```python
from build123d import *

# Parameters (mm, degrees)
F0_W     = 78.25
F0_H     = 40
F1_DEPTH = 2
F3_DEPTH = 77.25


with BuildPart() as f1:
    # F0 (on Top) → F1 (new body)
    with BuildSketch(Plane.XY):
        Rectangle(F0_W, F0_H)
    extrude(amount=F1_DEPTH)

    # F2 (on face) → F3 (cut)
    with BuildSketch(Plane(origin=(-39.125, 0, 0), x_dir=(0, -1, 0), z_dir=(-1, 0, 0))):
        Polygon((18, 2), (-18, 2), (-19, 0), (19, 0), align=None)
    extrude(amount=-F3_DEPTH, mode=Mode.SUBTRACT)


solid = f1.part
```
The listing builds one solid part. Answer for the finished solid, in the listing's coordinates (mm). A direction names the side the tool comes from. Give positions to 0.01 mm unless a question says otherwise; leave off trailing zeros. Order: outer loops, then holes, each group sorted by start corner. A loop starts at its lowest first (then second) coordinate and runs counter-clockwise, first axis right, second up. Notation, with made-up numbers: (20.5, 48.25) - (40.5, 48.25) arc R21 ccw to (40.5, 53.25) - close; hole circle Ø9 at (83, -28.5). An arc over 180 degrees is marked (long way). Answer in a Markdown table with one row per item. Add a question column.
Q1. For a pull along Y with two mould halves and no side action, classify faces 1 (the flat face through (38.125, 0, 1)), 2 (the flat face through (-1, -20, 1)), 3 (the flat face through (-0.2, 19.4, 0)), 4 (the flat face through (-1, -18.5, 1)) as released by +Y, released by -Y, zero draft, split by the parting line, or undercut.
Q2. The part is cut by section A-A (x = 6.5). Determine the outline of the cut face in (y, z).
Q3. Which of the six approach directions +Z, -Z, +X, -X, +Y, -Y give full straight-line access (tool end or side, diameter ignored) to faces 5 (the flat face through (-1, 18.5, 1)), 6 (the flat face through (-1, 20, 1))?
Q4. Find the intervals of material crossed by line 1 along X through (y, z) = (15.5, 1.7) (3 decimals); line 2 along Y through (x, z) = (-14, 1); line 3 along Y through (x, z) = (9, 0.6), in increasing order. Write a range as [from, to].
Q5. The part is cut by section B-B (z = 0.6). Determine the outline of the cut face in (x, y) (3 decimals), then the cut area to 3 significant figures.
Q6. The part is cut by section C-C (y = -4). Determine the outline of the cut face in (x, z) (3 decimals).
Determined:
| question | item | result |
|---|---|---|
| 1 | face 1 | undercut |
| 1 | face 2 | released by -Y |
| 1 | face 3 | zero draft |
| 1 | face 4 | undercut |
| 2 | outline | (-20, 0) - (-19, 0) - (-18, 2) - (-20, 2) - close; (18, 2) - (19, 0) - (20, 0) - (20, 2) - close |
| 3 | face 5 | -Z, -X |
| 3 | face 6 | +Z, -Z, +X, -X, +Y |
| 4 | line 1 | x = [38.125, 39.125] |
| 4 | line 2 | y = [-20, -18.5], [18.5, 20] |
| 4 | line 3 | y = [-20, -18.7], [18.7, 20] |
| 5 | outline | (-39.125, -20) - (39.125, -20) - (39.125, 20) - (-39.125, 20) - (-39.125, 18.7) - (38.125, 18.7) - (38.125, -18.7) - (-39.125, -18.7) - close |
| 5 | area | 241 mm² |
| 6 | outline | (38.125, 0) - (39.125, 0) - (39.125, 2) - (38.125, 2) - close |
